Input: part model. Units: mm. Frame: model coordinates. A direction names the side the tool comes from. Round coordinates to 2 decimals unless told otherwise and drop trailing zeros. Loops run counter-clockwise (first coordinate to the right, second up) from the corner with the lowest first, then second, coordinate; pieces in that order, holes last. Notation, with made-up numbers: M -13,72 L 16,72 A20 cw 16,106 Z; hole C 69,39.5 d6. An arc over 180 degrees is marked long. Return JSON: item names as keys, results as strings. Group by question number.
1) Mould query, pull axis X, two halves, no side actions, for faces 1 (the face through (10.736, -12.522, 0.258)), 2 (the face through (38, -25.4, -3)), 3 (the face through (61.536, -12.522, 0.258)), 4 (the face through (76.2, 0, 0)). Classes: +X half, -X half, draft (parallel to the pull), parting line (faces both ways), or undercut.
2) Contact query for a flat-ended pin moving along its axis: P1, Ø2.5, axis at x = 38.1, z = 0, coming from the -Y side. Output: stop coordinate, or through.
3) Section B-B (y = -9.5). Output: boundary loops of the cut face in (x, z).
4) Section A-A (z = 4). Output: boundary loops of the cut face in (x, y), plus the area to 3 significant figures.
5) Section C-C (x = 20). Output: boundary loops of the cut face in (y, z), plus the area to 3 significant figures.
6) Material intervals for line 1 (X direction, y = -20, z = 0); line 2 (Z direction, x = 38.1, y = -6.5); line 3 (Y direction, x = 19, z = 0), sorted ascending. Write a range as from..to.
7) Access query for faces 5 (the face through (40.034, -12.522, 0.429)), 6 (the face through (38, 25.4, 0)). Directions: +Z, -Z, +X, -X, +Y, -Y. A direction counts if a zero-diameter tool reaches every point of the face in a straight line with its end or side. Return the directions, or none.
Autodesk Inventor part; units mm, degrees
ref_plane "YZ Plane" through (0, 0, 0) normal (1, 0, 0) x (0, 1, 0)
ref_plane "XZ Plane" through (0, 0, 0) normal (0, 1, 0) x (-1, 0, 0)
ref_plane "XY Plane" through (0, 0, 0) normal (0, 0, 1) x (1, 0, 0)
sketch "Sketch1" plane through (0, 0, 0) normal (1, 0, 0) x (0, 1, 0)
  line L0 (25.4, 12.7) -> (-25.4, 12.7)
  line L1 (-25.4, 12.7) -> (-25.4, -12.7)
  line L2 (-25.4, -12.7) -> (25.4, -12.7)
  line L3 (25.4, -12.7) -> (25.4, 12.7)
  line L4 (25.4, 12.7) -> (-25.4, -12.7) construction
  line L5 (-25.4, 12.7) -> (25.4, -12.7) construction
  point P0 (0, 0)
  dimension "d0" = 50.8
  dimension "d1" = 25.4
extrude "Extrusion1" add sketch "Sketch1" along normal blind 76.2
sketch "Sketch2" plane through (76.2, 0, 0) normal (1, 0, 0) x (0, 0, -1)
  line L0 (12.7, 25.4) -> (-12.7, 25.4) construction
  point P0 (0, 0)
  point P1 (0, 12.7)
  dimension "d4" = 12.7
hole "Hole1" at (76.2, 12.7, 0) direction (-1, 0, 0) diameter 12.7 end through all
sketch "Sketch3" plane through (0, -25.4, -12.7) normal (0, -1, 0) x (1, 0, 0)
  line L0 (0, 0) -> (76.2, 0) construction
  line L1 (63.5, 12.7) -> (12.7, 12.7) construction
  line L2 (76.2, 25.4) -> (76.2, 0) construction
  point P0 (0, 12.7)
  point P1 (38.1, 12.7)
  point P2 (38.1, 0)
  point P3 (38.1, 12.7)
  point P4 (76.2, 12.7)
  dimension "d12" = 50.8
hole "Hole2" at (63.5, -25.4, 0) at (38.1, -25.4, 0) at (12.7, -25.4, 0) direction (0, 1, 0) diameter 3.9624 depth 25.4 tip angle 118
properties part number "CHD-001" material "Aluminum 6061"
Returned:
{
 "1": {"face 1": "undercut", "face 2": "draft", "face 3": "undercut", "face 4": "+X half"},
 "2": {"P1": "stops at y = 0.44"},
 "3": {"outline": "M 0,-12.7 L 76.2,-12.7 L 76.2,12.7 L 0,12.7 Z; hole C 12.7,0 d3.96; hole C 38.1,0 d3.96; hole C 63.5,0 d3.96"},
 "4": {"outline": "M 0,-25.4 L 76.2,-25.4 L 76.2,7.77 L 0,7.77 Z; M 0,17.63 L 76.2,17.63 L 76.2,25.4 L 0,25.4 Z", "area": "3,120 mm^2"},
 "5": {"outline": "M -25.4,-12.7 L 25.4,-12.7 L 25.4,12.7 L -25.4,12.7 Z; hole C 12.7,0 d12.7", "area": "1,160 mm^2"},
 "6": {"line 1": "x = 0..10.72, 14.68..36.12, 40.08..61.52, 65.48..76.2", "line 2": "z = -12.7..-1.98, 1.98..12.7", "line 3": "y = -25.4..6.35, 19.05..25.4"},
 "7": {"face 5": "-Y", "face 6": "+Z, -Z, +X, -X, +Y"}
}
